```python
from build123d import *

# Parameters (mm, degrees)
BOSS_EXTRUDE1_DEPTH = 39.878
SKETCH3_R           = 1.5875
CUT_EXTRUDE1_DEPTH  = 90.788257027
SKETCH5_W           = 5.295414823
SKETCH5_H           = 5.612914704
CUT_EXTRUDE2_DEPTH  = 124.157023236
SKETCH6_R           = 1.576757794
SKETCH6_R_2         = 1
SKETCH6_R_3         = 1.536946723
SKETCH6_R_4         = 1.574598992
SKETCH6_R_5         = 1.626931784
BOSS_EXTRUDE3_DEPTH = 2.54


with BuildPart() as part:
    # Sketch2 → Boss-Extrude1 (new body)
    with BuildSketch(Plane.XY):
        Polygon((-30.226, 0), (-30.226, -5.08), (-38.1, -5.08), (-38.1, 0), (-32.766, 0), (-32.766, 2.54), (-2.54, 2.54), (-2.54, 18.288), (66.310002, 18.288), (66.310002, 0), (76.978002, 0), (76.978002, -5.08), (65.040002, -5.08), (65.040002, 15.748), (0, 15.748), (0, 0), align=None)
    extrude(amount=BOSS_EXTRUDE1_DEPTH)

    # Sketch3 → Cut-Extrude1 (cut, through all)
    with BuildSketch(Plane.XZ.offset(5.08)):
        with Locations((-34.544, 12.369063527)):
            Circle(SKETCH3_R)
        with Locations((72.644, 12.369063527)):
            Circle(SKETCH3_R)
    extrude(amount=-CUT_EXTRUDE1_DEPTH, mode=Mode.SUBTRACT)

    # Sketch5 → Cut-Extrude2 (cut, through all)
    with BuildSketch(Plane(origin=(76.978002, 0, 0), x_dir=(0, 0, -1), z_dir=(1, 0, 0))):
        with Locations((-37.230292589, 15.481542648)):
            Rectangle(SKETCH5_W, SKETCH5_H)
    extrude(amount=-CUT_EXTRUDE2_DEPTH, mode=Mode.SUBTRACT)

    # Sketch6 → Boss-Extrude3 (add)
    # profile 1 of 4: a face of its own
    with BuildSketch(Plane(origin=(0, 2.54, 0), x_dir=(1, 0, 0), z_dir=(0, 1, 0))):
        with Locations((-29.54, -27.73004556)):
            Circle(SKETCH6_R)
        with Locations(Location((-29.54, -27.73004556, 0), (0, 0, 180))):
            Circle(SKETCH6_R_2, mode=Mode.SUBTRACT)
    # profile 2 of 4: a face of its own
    with BuildSketch(Plane(origin=(0, 2.54, 0), x_dir=(1, 0, 0), z_dir=(0, 1, 0))):
        with Locations((-29.54, -2.73004556)):
            Circle(SKETCH6_R_3)
        with Locations(Location((-29.54, -2.73004556, 0), (0, 0, 180))):
            Circle(SKETCH6_R_2, mode=Mode.SUBTRACT)
    # profile 3 of 4: a face of its own
    with BuildSketch(Plane(origin=(0, 2.54, 0), x_dir=(1, 0, 0), z_dir=(0, 1, 0))):
        with Locations((-4.54, -27.73004556)):
            Circle(SKETCH6_R_4)
        with Locations(Location((-4.54, -27.73004556, 0), (0, 0, 180))):
            Circle(SKETCH6_R_2, mode=Mode.SUBTRACT)
    # profile 4 of 4: a face of its own
    with BuildSketch(Plane(origin=(0, 2.54, 0), x_dir=(1, 0, 0), z_dir=(0, 1, 0))):
        with Locations((-4.54, -2.73004556)):
            Circle(SKETCH6_R_5)
        with Locations(Location((-4.54, -2.73004556, 0), (0, 0, 180))):
            Circle(SKETCH6_R_2, mode=Mode.SUBTRACT)
    extrude(amount=BOSS_EXTRUDE3_DEPTH)


solid = part.part
```
Can you work these out from the model? Positions are in its coordinate system, mm. A direction names the side the tool comes from. Coordinates: 2 decimals unless noted, no trailing zeros. Write each loop counter-clockwise with the first axis right and the second up, starting at its lowest first coordinate (ties: lowest second). Pieces come first, ordered by that corner, then holes. Notation, with made-up numbers: M 12.5,64 L 55.5,64 A34 cw 55.5,97 Z; hole C 78.5,-19 d7. An arc over 180 degrees is marked long. Answer as CSV lines item,"result".
Item 1: Imagine slicing it at D-D on x = -4.54. List the corners of the cut face in (y, z) for me, plus the area to 3 significant figures.
Geometry results:
outline,"M 0,0 L 2.54,0 L 2.54,1.1 L 5.08,1.1 L 5.08,1.73 L 2.54,1.73 L 2.54,3.73 L 5.08,3.73 L 5.08,4.36 L 2.54,4.36 L 2.54,26.16 L 5.08,26.16 L 5.08,26.73 L 2.54,26.73 L 2.54,28.73 L 5.08,28.73 L 5.08,29.3 L 2.54,29.3 L 2.54,39.88 L 0,39.88 Z"
area,"107 mm2"
Item 2: Imagine slicing it at B-B on y = -3. List the corners of the cut face in (x, z) for me (1 decimal), plus the area to 3 significant figures.
Geometry results:
outline,"M -38.1,0 L -30.2,0 L -30.2,39.9 L -38.1,39.9 Z; M 65,0 L 77,0 L 77,39.9 L 65,39.9 Z; hole C -34.5,12.4 d3.2; hole C 72.6,12.4 d3.2"
area,"774 mm2"
Item 3: We'd pull the mould along X, two halves only. Please class faces 5 (the flat face through (-19, 1, 39.878)), 6 (the flat face through (-38.1, -3, 20)), 7 (the flat face through (-30, 2.54, 28)): +X half, -X half, draft (parallel to the pull), parting line (faces both ways), or undercut.
Geometry results:
face 5,"draft"
face 6,"-X half"
face 7,"undercut"
Item 4: Please list where these lines run through material, in increasing order: line 1 along Z through (x, y) = (-29.54, 3.9); line 2 along Z through (x, y) = (-4.54, 3.2); line 3 along X through (y, z) = (15.5, 28.5).
Geometry results:
line 1,"z = 1.19 to 1.73, 3.73 to 4.27, 26.15 to 26.73, 28.73 to 29.31"
line 2,"z = 1.1 to 1.73, 3.73 to 4.36, 26.16 to 26.73, 28.73 to 29.3"
line 3,"x = -2.54 to 0, 65.04 to 66.31"
Item 5: Imagine slicing it at A-A on z = 37.5. List the corners of the cut face in (x, y) for me, plus the area to 3 significant figures.
Geometry results:
outline,"M -38.1,-5.08 L -30.23,-5.08 L -30.23,0 L 0,0 L 0,12.68 L -2.54,12.68 L -2.54,2.54 L -32.77,2.54 L -32.77,0 L -38.1,0 Z; M 65.04,-5.08 L 76.98,-5.08 L 76.98,0 L 66.31,0 L 66.31,12.68 L 65.04,12.68 Z"
area,"226 mm2"
Item 6: On a 3-axis mill with a long thin cutter (end or side, diameter ignored), from which of +Z, -Z, +X, -X, +Y, -Y can I reach the whole of each face in a straight line? I mean faces 1 (the flat face through (-30, 5.08, 29)), 2 (the flat face through (-30, 2.54, 3)), 3 (the flat face through (72, 0, 20)), 4 (the flat face through (33, 15.748, 17)). Say none if no direction works.
Geometry results:
face 1,"+Z, -Z, -X, +Y"
face 2,"+Y"
face 3,"+Z, -Z, +X, +Y"
face 4,"+Z, -Z, -Y"
Item 7: Imagine slicing it at C-C on z = 23. List the corners of the cut face in (x, y) for me.
Geometry results:
outline,"M -38.1,-5.08 L -30.23,-5.08 L -30.23,0 L 0,0 L 0,15.75 L 65.04,15.75 L 65.04,-5.08 L 76.98,-5.08 L 76.98,0 L 66.31,0 L 66.31,18.29 L -2.54,18.29 L -2.54,2.54 L -32.77,2.54 L -32.77,0 L -38.1,0 Z"
Item 8: I'm going to push flat-ended pins straight in: P1, Ø1.3, axis at x = -1.5, z = 36, coming from the +Y side; P2, Ø12, axis at x = 55, z = 34, coming from the -Y side; P3, Ø9, axis at x = -23.5, z = 13.5, coming from the +Y side; P4, Ø2, axis at x = 0.5, y = 1, coming from the +Z side. Where does each tip first touch, or does it pass through?
Geometry results:
P1,"stops at y = 12.68"
P2,"stops at y = 15.75"
P3,"stops at y = 2.54"
P4,"stops at z = 39.88"
